Geometry: final body of the model. Coordinates: model frame, mm. Round coordinates to 2 decimals unless told otherwise and drop trailing zeros. Loops run counter-clockwise (first coordinate to the right, second up) from the corner with the lowest first, then second, coordinate; pieces in that order, holes last. Notation, with made-up numbers: M 87.5,49 L 95.5,49 A21 cw 95.5,73 Z; hole C 23.5,11 d6. An arc over 180 degrees is marked long. Write each question's results on one line, items separated by ' | '.
Autodesk Inventor part; units mm, degrees
ref_plane "YZ Plane" through (0, 0, 0) normal (1, 0, 0) x (0, 1, 0)
ref_plane "XZ Plane" through (0, 0, 0) normal (0, 1, 0) x (-1, 0, 0)
ref_plane "XY Plane" through (0, 0, 0) normal (0, 0, 1) x (1, 0, 0)
sketch "Náčrt1" plane through (0, 0, 0) normal (0, 0, 1) x (1, 0, 0)
  line L0 (0, 7.375) -> (0, -7.375) construction
  line L1 (-3.5, 7.375) -> (-3.5, -7.375)
  line L2 (3.5, -7.375) -> (3.5, 7.375)
  arc A0 (3.5, 7.375) -> (-3.5, 7.375) centre (0, 7.375) ccw
  arc A1 (-3.5, -7.375) -> (3.5, -7.375) centre (0, -7.375) ccw
  circle A2 centre (0, 7.375) radius 1.7
  circle A3 centre (0, -7.375) radius 1.7
  circle A4 centre (0, 7.375) radius 3.5
  point P0 (0, 0)
  point P1 (0, 0)
  point P2 (-3.5, 7.375)
  point P3 (3.5, 7.375)
  dimension "d0" = 14.75
  dimension "d1" = 3.5
  dimension "d2" = 3.4
extrude "Vysunutí1" add sketch "Náčrt1" along normal blind 1.2
properties part number "not flex back qre flex holder"
1. Section C-C (x = 1.5). Output: boundary loops of the cut face in (y, z) (3 decimals).
Answer key:
outline: M -10.537,0 L -8.175,0 L -8.175,1.2 L -10.537,1.2 Z; M -6.575,0 L 6.575,0 L 6.575,1.2 L -6.575,1.2 Z; M 8.175,0 L 10.537,0 L 10.537,1.2 L 8.175,1.2 Z
2. Section B-B (z = 0.75). Output: boundary loops of the cut face in (x, y) (3 decimals).
Answer key:
outline: M -3.5,-7.375 A3.5 ccw 3.5,-7.375 L 3.5,7.375 A3.5 ccw -3.5,7.375 Z; hole C 0,-7.375 d3.4; hole C 0,7.375 d3.4
3. Section D-D (x = -2). Output: boundary loops of the cut face in (y, z), then the cut area to 3 significant figures.
Answer key:
outline: M -10.25,0 L 10.25,0 L 10.25,1.2 L -10.25,1.2 Z | area: 24.6 mm²
4. Section A-A (x = 0). Output: boundary loops of the cut face in (y, z) (3 decimals), then the cut area to 3 significant figures.
Answer key:
outline: M -10.875,0 L -9.075,0 L -9.075,1.2 L -10.875,1.2 Z; M -5.675,0 L 5.675,0 L 5.675,1.2 L -5.675,1.2 Z; M 9.075,0 L 10.875,0 L 10.875,1.2 L 9.075,1.2 Z | area: 17.9 mm²
5. Ray query, probe 1 along Y at (x, z) = (0, 0.75) (3 decimals); probe 2 along Y at (x, z) = (1.25, 1); probe 3 along X at (y, z) = (7.75, 0.1). Return the intervals inside material, ascending.
Answer key:
probe 1: y = -10.875 to -9.075, -5.675 to 5.675, 9.075 to 10.875 | probe 2: y = -10.64 to -8.53, -6.22 to 6.22, 8.53 to 10.64 | probe 3: x = -3.48 to -1.66, 1.66 to 3.48
6. Draft query along X for faces 1 (the face through (-0.369, 9.035, 0.592)), 2 (the face through (-3.5, 0, 1)), 3 (the face through (-0.077, 10.874, 0.592)), 4 (the face through (0, 0, 0)). Return one class per face: pulls with the +X half, pulls with the -X half, needs draft (parallel to the pull), parting line crosses it, or undercut.
Answer key:
face 1: undercut | face 2: pulls with the -X half | face 3: parting line crosses it | face 4: needs draft
